Geometry check sheet. Reference: the model listing, model coordinates, mm. Face numbers are marked on the shaded views. A direction names the side the tool comes from. Round coordinates to 2 decimals unless told otherwise and drop trailing zeros. Loops run counter-clockwise (first coordinate to the right, second up) from the corner with the lowest first, then second, coordinate; pieces in that order, holes last. Notation, with made-up numbers: (-38, -15) - (14, -15) arc R37 ccw to (14, 22) - close; hole circle Ø9 at (84.25, 44). An arc over 180 degrees is marked (long way). Answer as CSV lines item,"result". Start each with the question number.
1) Cross-section at A-A on z = 9.25. Record the boundary of the cut face in (x, y), and give its area (3 significant figures).
2) Cross-section at B-B on y = -3. Record the boundary of the cut face in (x, z), and give its area (3 significant figures).
3) Cross-section at C-C on x = 76. Record the boundary of the cut face in (y, z), and give its area (3 significant figures).
4) Cross-section at D-D on z = 0. State how many separate pieces and enclosed holes the cut face has, and give its area (3 significant figures).
5) Depth check by flat-ended pin: P1, Ø4, axis at y = -11, z = -6, coming from the -X side; P2, Ø7, axis at y = 0, z = -5.5, coming from the +X side; P3, Ø10, axis at x = 4.5, z = -1, coming from the +Y side. Enter the tip coordinate at first touch or a pass-through.
6) Thickness scan on line 1 along X through (y, z) = (16.1, 0); line 2 along Y through (x, z) = (124, -3.75); line 3 along X through (y, z) = (-4, 5.5). Record the ranges inside material, lowest first.
7) Access from +Z, -Z, +X, -X, +Y, -Y to the whole of each face (thin tool, end or side, straight path). Record for the marked faces 4, 5, 6, 7 and 8.
8) Draft check along X on the marked faces 1, 2 and 3. Enter one of: released by +X, released by -X, zero draft, split by the parting line, or undercut.
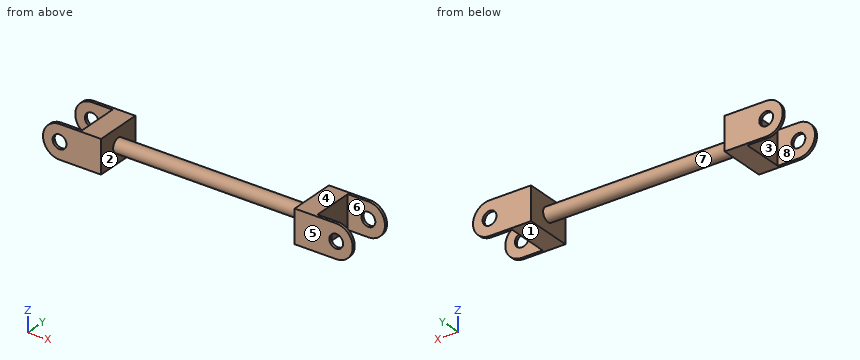
from build123d import *

# Parameters (mm, degrees)
BOSS_EXTRUDE1_DEPTH        = 17
BOSS_EXTRUDE1_DEPTH_BACK   = 17
SKETCH1_R                  = 5
BOSS_EXTRUDE1_2_DEPTH      = 17
BOSS_EXTRUDE1_2_DEPTH_BACK = 17
SKETCH3_R                  = 5
BOSS_EXTRUDE2_DEPTH        = 140
CUT_EXTRUDE1_DEPTH         = 15
CUT_EXTRUDE1_DEPTH_BACK    = 15


with BuildPart() as part:
    # Sketch1 → Boss-Extrude1 (new, two sides: drawn at the far end of the back side and taken through both)
    with BuildSketch(Plane(origin=(0, 0, 0), x_dir=(1, 0, 0), z_dir=(0, 1, 0)).offset(-BOSS_EXTRUDE1_DEPTH_BACK)):
        with BuildLine():
            Line((-69.176769869, 12), (-39.176769869, 12))
            Line((-39.176769869, 12), (-39.176769869, -12))
            Line((-39.176769869, -12), (-69.176769869, -12))
            ThreePointArc((-69.176769869, -12), (-81.176769869, 0), (-69.176769869, 12))
        make_face()
        with Locations(Location((-69.176769869, 0, 0), (0, 0, 270))):
            Circle(SKETCH1_R, mode=Mode.SUBTRACT)
    extrude(amount=BOSS_EXTRUDE1_DEPTH + BOSS_EXTRUDE1_DEPTH_BACK)



with BuildPart() as body_2:
    # Sketch1 → Boss-Extrude1 2 (new, two sides: drawn at the far end of the back side and taken through both)
    with BuildSketch(Plane(origin=(0, 0, 0), x_dir=(1, 0, 0), z_dir=(0, 1, 0)).offset(-BOSS_EXTRUDE1_2_DEPTH_BACK)):
        with BuildLine():
            Line((130.823230131, 12), (100.823230131, 12))
            Line((100.823230131, 12), (100.823230131, -12))
            Line((100.823230131, -12), (130.823230131, -12))
            ThreePointArc((130.823230131, -12), (142.823230131, 0), (130.823230131, 12))
        make_face()
        with Locations(Location((130.823230131, 0, 0), (0, 0, 270))):
            Circle(SKETCH1_R, mode=Mode.SUBTRACT)
    extrude(amount=BOSS_EXTRUDE1_2_DEPTH + BOSS_EXTRUDE1_2_DEPTH_BACK)


with BuildPart() as part_1:
    add(part.part)

    add(body_2.part)  # Boss-Extrude2 merges body 2
    # Sketch3 → Boss-Extrude2 (add)
    with BuildSketch(Plane(origin=(-39.176769869, 0, 0), x_dir=(0, 0, -1), z_dir=(1, 0, 0))):
        with Locations(Location((0, 0, 0), (0, 0, 180))):
            Circle(SKETCH3_R)
    extrude(amount=BOSS_EXTRUDE2_DEPTH)

    # Sketch4 → Cut-Extrude1 (cut, two sides: drawn at the far end of the back side and taken through both)
    with BuildSketch(Plane(origin=(0, 0, 0), x_dir=(1, 0, 0), z_dir=(0, 1, 0)).offset(-CUT_EXTRUDE1_DEPTH_BACK)):
        with BuildLine():
            Line((115.823230131, -12), (130.823230131, -12))
            ThreePointArc((130.823230131, -12), (142.823230131, 0), (130.823230131, 12))
            Line((130.823230131, 12), (115.823230131, 12))
            Line((115.823230131, 12), (115.823230131, -12))
        make_face()
        with BuildLine():
            Line((-69.176769869, -12), (-54.176769869, -12))
            Line((-54.176769869, -12), (-54.176769869, 12))
            Line((-54.176769869, 12), (-69.176769869, 12))
            ThreePointArc((-69.176769869, 12), (-81.176769869, 0), (-69.176769869, -12))
        make_face()
    extrude(amount=CUT_EXTRUDE1_DEPTH + CUT_EXTRUDE1_DEPTH_BACK, mode=Mode.SUBTRACT)


solid = part_1.part
Answer block:
1,outline,"(-76.82, -17) - (-39.18, -17) - (-39.18, 17) - (-76.82, 17) - (-76.82, 15) - (-54.18, 15) - (-54.18, -15) - (-76.82, -15) - close; (100.82, -17) - (138.47, -17) - (138.47, -15) - (115.82, -15) - (115.82, 15) - (138.47, 15) - (138.47, 17) - (100.82, 17) - close"
1,area,"1,200 mm^2"
2,outline,"(-54.18, -12) - (-39.18, -12) - (-39.18, -4) - (100.82, -4) - (100.82, -12) - (115.82, -12) - (115.82, 12) - (100.82, 12) - (100.82, 4) - (-39.18, 4) - (-39.18, 12) - (-54.18, 12) - close"
2,area,"1,840 mm^2"
3,outline,"circle Ø10 at (0, 0)"
3,area,"78.5 mm^2"
4,separate pieces,"5"
4,enclosed holes,"0"
4,area,"2,560 mm^2"
5,P1,"stops at x = -54.18"
5,P2,"stops at x = 115.82"
5,P3,"stops at y = 5"
6,line 1,"x = -81.18 to -74.18, -64.18 to -39.18, 100.82 to 125.82, 135.82 to 142.82"
6,line 2,"y = -17 to -15, 15 to 17"
6,line 3,"x = -54.18 to -39.18, 100.82 to 115.82"
7,face 4,"+Z, +X, -X, +Y, -Y"
7,face 5,"+Z, -Z, +X, -X, -Y"
7,face 6,"+Z, -Z, +X"
7,face 7,"none"
7,face 8,"+Z, -Z, -X"
8,face 1,"zero draft"
8,face 2,"undercut"
8,face 3,"released by -X"
